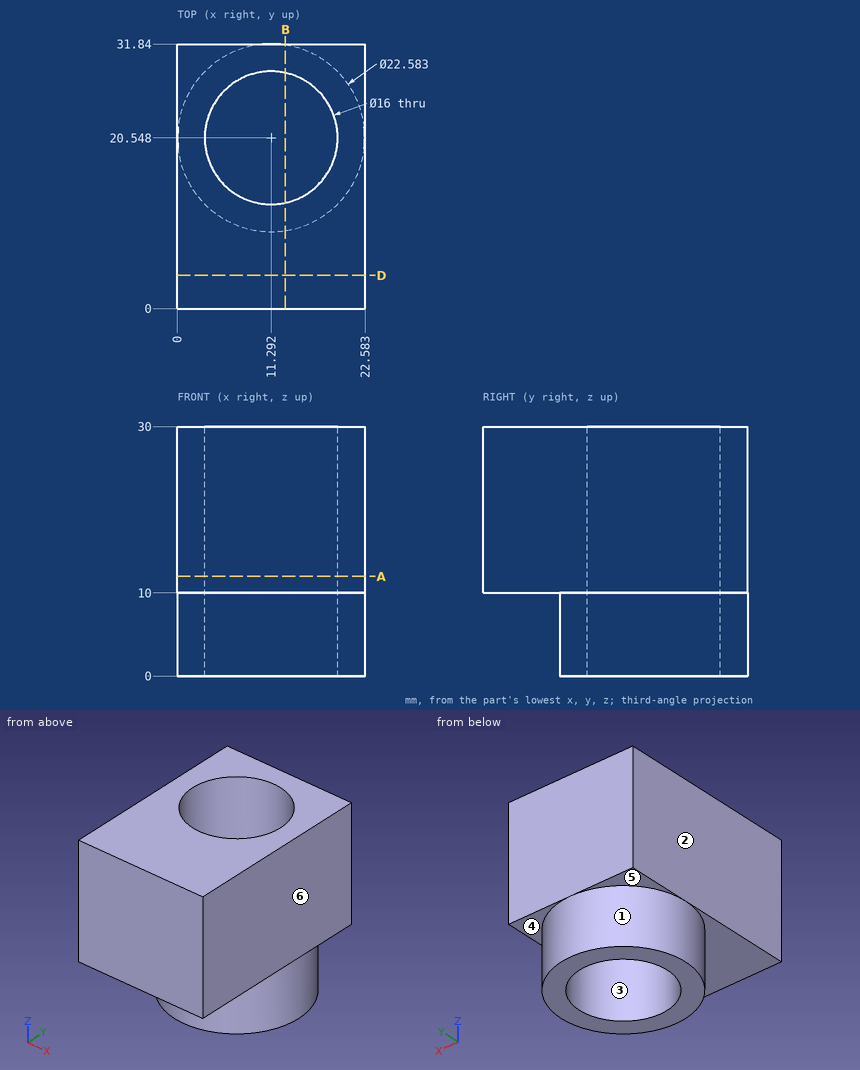
Check sheet for the drawn part. Datum: minimum x, y, z corner. Units: mm. A direction names the side the tool comes from. Round coordinates to 2 decimals unless told otherwise and drop trailing zeros. Loops run counter-clockwise (first coordinate to the right, second up) from the corner with the lowest first, then second, coordinate; pieces in that order, holes last. Notation, with made-up numbers: (14, -1) -> (47, -1) arc R33 cw to (47, 32) -> close; hole circle Ø8 at (83.25, -21.5). An arc over 180 degrees is marked (long way). Put each result on its own line as item: value. Start each with the question number.
1. Gauge pin test, flat ends, axial feed: pin 1 (4 mm diameter, centred on x = 10.5, y = 4.5, fed in from -Z); pin 2 (4 mm diameter, centred on y = 4, z = 7.5, fed in from +X). Record the tip position at first contact, or that the pin passes through.
2. Scan lines: probe 1 along Y at (x, z) = (16.75, 18.5) (1 decimal); probe 2 along Y at (x, z) = (7.75, 16.75) (1 decimal); probe 3 along Z at (x, y) = (2, 9.5). Record each from-to range of solid material in increasing order.
3. Access from +Z, -Z, +X, -X, +Y, -Y to the whole of each face (thin tool, end or side, straight path). Record for the marked faces 5 and 6.
4. Draft check along X on the marked faces 1, 2, 3 and 4. Enter one of: +X half, -X half, draft (parallel to the pull), parting line (faces both ways), or undercut.
5. Section check B-B (x = 13). Enter the section's corners in (y, z).
6. Section check D-D (y = 4). Enter the section's corners in (x, z), plus the area to 3 significant figures.
7. Section check A-A (z = 12). Enter the section's corners in (x, y).
Findings:
1. pin 1: stops at z = 10
1. pin 2: passes through
2. probe 1: y = 0 to 14.7, 26.4 to 31.8
2. probe 2: y = 0 to 13.4, 27.7 to 31.8
2. probe 3: z = 10 to 30
3. face 5: -Z, -X, +Y
3. face 6: +Z, -Z, +X, +Y, -Y
4. face 1: parting line
4. face 2: -X half
4. face 3: undercut
4. face 4: draft
5. outline: (0, 10) -> (9.39, 10) -> (9.39, 0) -> (12.73, 0) -> (12.73, 30) -> (0, 30) -> close; (28.36, 0) -> (31.71, 0) -> (31.71, 10) -> (31.84, 10) -> (31.84, 30) -> (28.36, 30) -> close
6. outline: (0, 10) -> (22.58, 10) -> (22.58, 30) -> (0, 30) -> close
6. area: 452 mm^2
7. outline: (0, 0) -> (22.58, 0) -> (22.58, 31.84) -> (0, 31.84) -> close; hole circle Ø16 at (11.29, 20.55)
